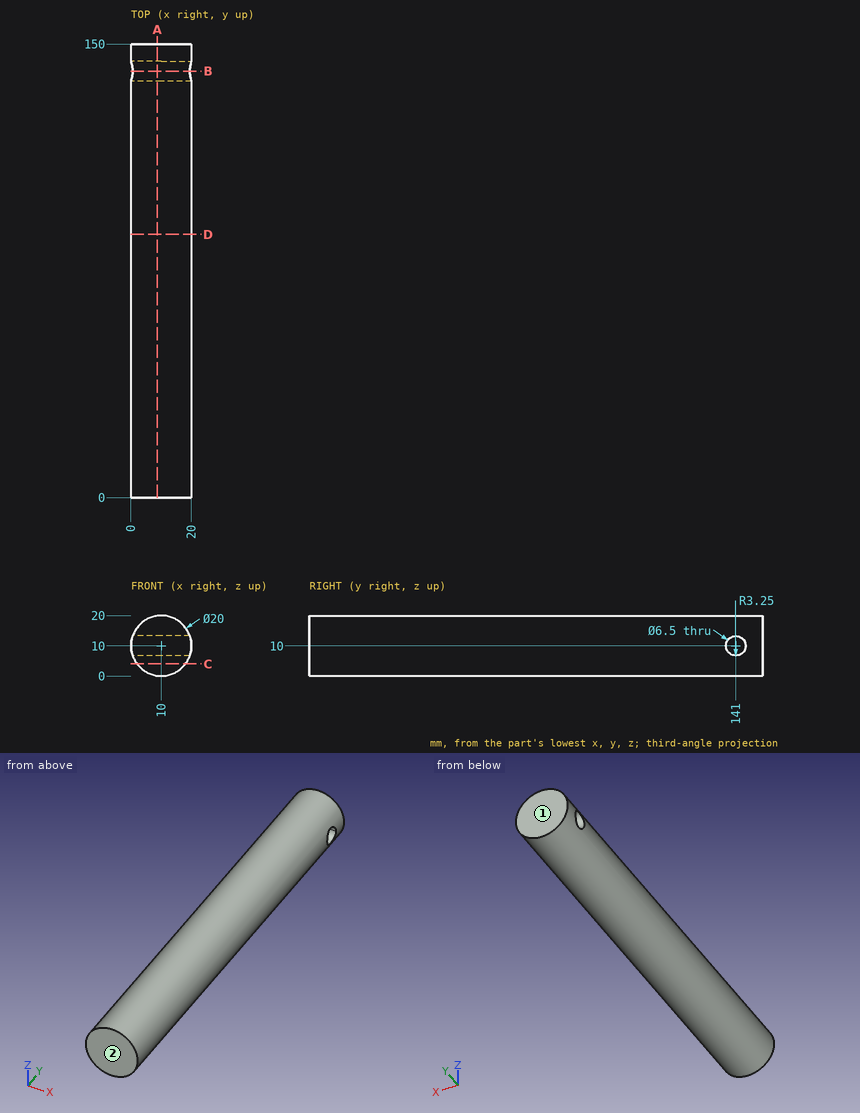
Part print with two shaded views. Sizes in mm from the minimum x, y, z corner. Round coordinates to 2 decimals unless told otherwise and drop trailing zeros. Order: outer loops, then holes, each group sorted by start corner. A loop starts at its lowest first (then second) coordinate and runs counter-clockwise, first axis right, second up. Notation, with made-up numbers: (-36.5, 22.25) - (-8.5, 22.25) arc R14 cw to (-8.5, 39.25) - close; hole circle Ø3 at (-32, 77). An arc over 180 degrees is marked (long way). Answer in a Markdown table with one row per item. Add a question column.
(1) Band-saw the part on C-C on z = 4. List the corners of the cut face in (x, y).
(2) Band-saw the part on A-A on x = 8.75. List the corners of the cut face in (y, z), and give its area (3 significant figures).
(3) Mould opens along Y. For the marked faces 1 and 2 say: +Y half, -Y half, draft (parallel to the pull), parting line (faces both ways), or undercut.
(4) Probe L1, parallel to Z at x = 10.5, y = 115; L2, parallel to Z at x = 7.25, y = 141; L3, parallel to Z at x = 9, y = 50. List the from-to ranges inside material, lowest first. Write a range as [from, to].
(5) Band-saw the part on D-D on y = 87. List the corners of the cut face in (x, z), and give its area (3 significant figures).
(6) Band-saw the part on B-B on y = 141. List the corners of the cut face in (x, z), and give its area (3 significant figures).
(7) Drop flat-ended pins along their axis: pin 1 Ø2 at (y, z) = (95, 15) entering from -X; pin 2 Ø10 at (x, y) = (2, 79) entering from -Z; pin 3 Ø8.5 at (y, z) = (141, 10) entering from -X; pin 4 Ø4 at (x, y) = (15.5, 85.5) entering from +Z. Give the stop position or say it passes through.
Data:
| question | item | result |
|---|---|---|
| 1 | outline | (2, 0) - (18, 0) - (18, 150) - (2, 150) - close |
| 2 | outline | (0, 0.08) - (150, 0.08) - (150, 19.92) - (0, 19.92) - close; hole circle Ø6.5 at (141, 10) |
| 2 | area | 2,940 mm^2 |
| 3 | face 1 | +Y half |
| 3 | face 2 | -Y half |
| 4 | L1 | z = [0.01, 19.99] |
| 4 | L2 | z = [0.39, 6.75], [13.25, 19.61] |
| 4 | L3 | z = [0.05, 19.95] |
| 5 | outline | circle Ø20 at (10, 10) |
| 5 | area | 314 mm^2 |
| 6 | outline | (0.54, 6.75) arc R10 ccw to (19.46, 6.75) - close; (0.54, 13.25) - (19.46, 13.25) arc R10 ccw to start |
| 6 | area | 186 mm^2 |
| 7 | pin 1 | stops at x = 0.83 |
| 7 | pin 2 | stops at z = 0.46 |
| 7 | pin 3 | stops at x = 0 |
| 7 | pin 4 | stops at z = 19.37 |
